Here's how the part is built. I have some questions about the finished solid (model axes, mm). Give positions to 0.01 mm unless a question says otherwise; leave off trailing zeros. Write each loop counter-clockwise with the first axis right and the second up, starting at its lowest first coordinate (ties: lowest second). Pieces come first, ordered by that corner, then holes. Notation, with made-up numbers: M -16,0 L 39,0 A26 ccw 39,27 Z; hole C 44,75 d7. An arc over 180 degrees is marked long. Answer as CSV lines item,"result". Start each with the question number.
Q1. Thinking about a two-plate mould opening in X: for faces 1 (the flat face through (0, -19.05, 0)), 2 (the cylindrical face through (4.38, -8.43, -0.04)), 3 (the flat face through (25.95, 0, 0)), which applies, +X half, -X half, draft (parallel to the pull), parting line (faces both ways), or undercut?
Q2. If I drill on line 1 along Y through (x, z) = (0, 0.95); line 2 along Y through (x, z) = (-6, -1.35); line 3 along X through (y, z) = (-2, -1.2), over which ranges is the centre line in solid material (lowest first)?
Q3. Suppose I cut it at C-C (y = -7.5). Write out the boundary of the cut face in (x, z).
Q4. Suppose I cut it at B-B (z = -0.9). Write out the boundary of the cut face in (x, y), then the cut area to 3 significant figures.
Q5. Suppose I cut it at A-A (x = 0). Write out the boundary of the cut face in (y, z).
```python
from build123d import *

# Parameters (mm, degrees)
F0_W     = 51.9
F0_H     = 38.1
F0_R     = 9.5
F1_DEPTH = 2.5


with BuildPart() as f1:
    # F0 (on Top) → F1 (new body, symmetric)
    with BuildSketch(Plane.XY):
        Rectangle(F0_W, F0_H)
        Circle(F0_R, mode=Mode.SUBTRACT)
    extrude(amount=F1_DEPTH, both=True)

    # F2 (on face) → F3 (revolve, cut)
    with BuildSketch(Plane.XY.offset(2.5)):
        with BuildLine():
            Line((14.65, -3.6893317878), (12.1541903113, -3.6755036277))
            ThreePointArc((12.1541903113, -3.6755036277), (11.7305653131, -4.8608133553), (11.1916659396, -5.9983566531))
            ThreePointArc((11.1916659396, -5.9983566531), (13.5381939434, -5.768494498), (14.65, -3.6893317878))
        make_face()
        with BuildLine():
            ThreePointArc((11.1916659396, -5.9983566531), (11.7305653131, -4.8608133553), (12.1541903113, -3.6755036277))
            Line((12.1541903113, -3.6755036277), (9.6501534838, -3.6616298846))
            ThreePointArc((9.6501534838, -3.6616298846), (10.0631779609, -5.0659848949), (11.1916659396, -5.9983566531))
        make_face()
    revolve(axis=Axis((12.1500767419, -3.6754808362, 2.5), (0.9999846515, -0.0055404657, 0)), mode=Mode.SUBTRACT)


solid = f1.part
```
Resolved:
1,face 1,"draft"
1,face 2,"undercut"
1,face 3,"+X half"
2,line 1,"-19.05 to -9.5, 9.5 to 19.05"
2,line 2,"-19.05 to -7.37, 7.37 to 19.05"
2,line 3,"-25.95 to -9.29, 9.29 to 25.95"
3,outline,"M -25.95,-2.5 L -5.83,-2.5 L -5.83,2.5 L -25.95,2.5 Z; M 5.83,-2.5 L 25.95,-2.5 L 25.95,2.5 L 5.83,2.5 Z"
4,outline,"M -25.95,-19.05 L 25.95,-19.05 L 25.95,19.05 L -25.95,19.05 Z; hole C 0,0 d19"
4,area,"1,690 mm^2"
5,outline,"M -19.05,-2.5 L -9.5,-2.5 L -9.5,2.5 L -19.05,2.5 Z; M 9.5,-2.5 L 19.05,-2.5 L 19.05,2.5 L 9.5,2.5 Z"
